Check sheet for the modelled part. Datum: model origin and axes. Units: mm. Give positions to 0.01 mm unless a question says otherwise; leave off trailing zeros. Order: outer loops, then holes, each group sorted by start corner. A loop starts at its lowest first (then second) coordinate and runs counter-clockwise, first axis right, second up.
Item 1: Material ranges on line 1 along Z through (x, y) = (-60, 7); line 2 along X through (y, z) = (7.5, -4); line 3 along Z through (x, y) = (47.5, 5.25), recorded low to high.
Item 2: Release check for a two-part mould opening along Z. For faces 1 (the flat face through (-3, 12, 0)), 2 (the cylindrical face through (-147.47, 6.08, 1.61)), 3 (the flat face through (-3, 6, -20)) record: released by +Z, released by -Z, zero draft, split by the parting line, or undercut.
Item 3: Sectioned sample at A-A on x = -135. Record the boundary of the cut face in (y, z), and give its area (3 significant figures).
Item 4: Sectioned sample at B-B on y = 9.75. Count the separate pieces of the cut face and the enclosed holes in it, and give its area (3 significant figures).
from build123d import *

# Parameters (mm, degrees)
SKETCH1_W           = 360
SKETCH1_H           = 40
BOSS_EXTRUDE1_DEPTH = 12
CUT_EXTRUDE1_REACH  = 183.505
SKETCH2_R           = 3
SKETCH2_R_2         = 5
LPATTERN1_COUNT     = 4
LPATTERN1_PITCH     = 90


with BuildPart() as part:
    # Sketch1 → Boss-Extrude1 (new body)
    with BuildSketch(Plane(origin=(0, 0, 0), x_dir=(1, 0, 0), z_dir=(0, 1, 0))):
        Rectangle(SKETCH1_W, SKETCH1_H)
    extrude(amount=BOSS_EXTRUDE1_DEPTH)

    # Sketch2 → Cut-Extrude1 (cut, up to next)
    with BuildSketch(Plane(origin=(0, 12, 0), x_dir=(1, 0, 0), z_dir=(0, 1, 0)), mode=Mode.PRIVATE) as cut_extrude1_sk1:
        with Locations(Location((-150, 0, 0), (0, 0, 270))):
            Circle(SKETCH2_R)
    cut_extrude1_tool1 = extrude(cut_extrude1_sk1.sketch, amount=-CUT_EXTRUDE1_REACH, mode=Mode.PRIVATE) & part.part
    # Sketch2 → Cut-Extrude1 (cut, up to next)
    with BuildSketch(Plane(origin=(0, 12, 0), x_dir=(1, 0, 0), z_dir=(0, 1, 0)), mode=Mode.PRIVATE) as cut_extrude1_sk2:
        with Locations(Location((-120, 0, 0), (0, 0, 270))):
            Circle(SKETCH2_R)
    cut_extrude1_tool2 = extrude(cut_extrude1_sk2.sketch, amount=-CUT_EXTRUDE1_REACH, mode=Mode.PRIVATE) & part.part
    # Sketch2 → Cut-Extrude1 (cut, up to next)
    with BuildSketch(Plane(origin=(0, 12, 0), x_dir=(1, 0, 0), z_dir=(0, 1, 0)), mode=Mode.PRIVATE) as cut_extrude1_sk3:
        with Locations(Location((-135, 0, 0), (0, 0, 270))):
            Circle(SKETCH2_R_2)
    cut_extrude1_tool3 = extrude(cut_extrude1_sk3.sketch, amount=-CUT_EXTRUDE1_REACH, mode=Mode.PRIVATE) & part.part
    cut_extrude1_1 = cut_extrude1_tool1.solids().sort_by_distance((-150, 12, 0))[0]
    add(cut_extrude1_1, mode=Mode.SUBTRACT)
    cut_extrude1_2 = cut_extrude1_tool2.solids().sort_by_distance((-120, 12, 0))[0]
    add(cut_extrude1_2, mode=Mode.SUBTRACT)
    cut_extrude1_3 = cut_extrude1_tool3.solids().sort_by_distance((-135, 12, 0))[0]
    add(cut_extrude1_3, mode=Mode.SUBTRACT)
    cut_extrude1 = cut_extrude1_1 + cut_extrude1_2 + cut_extrude1_3  # Cut-Extrude1 as one shape, for the pattern or mirror that repeats it

    # LPattern1: Cut-Extrude1 ×4
    with Locations(*[(i * LPATTERN1_PITCH, 0, 0) for i in range(1, LPATTERN1_COUNT)]):
        add(cut_extrude1, mode=Mode.SUBTRACT)


solid = part.part
Report:
1. line 1: z = -20 to -3, 3 to 20
1. line 2: x = -180 to -138, -132 to -48, -42 to 42, 48 to 132, 138 to 180
1. line 3: z = -20 to -4.33, 4.33 to 20
2. face 1: zero draft
2. face 2: undercut
2. face 3: released by -Z
3. outline: (0, -20) - (12, -20) - (12, -5) - (0, -5) - close; (0, 5) - (12, 5) - (12, 20) - (0, 20) - close
3. area: 360 mm2
4. separate pieces: 1
4. enclosed holes: 12
4. area: 13,900 mm2
